Model file for the job. Use its own axes, mm. Face numbers are marked on the shaded views. Coordinates: 2 decimals unless noted, no trailing zeros. Loops run counter-clockwise (first coordinate to the right, second up) from the corner with the lowest first, then second, coordinate; pieces in that order, holes last.
from build123d import *

# Parameters (mm, degrees)
F0_W     = 20
F0_H     = 10.1
F1_DEPTH = 1.5
F2_R     = 1.1
F3_DEPTH = 1.5
F4_R     = 1


with BuildPart() as f1:
    # F0 (on Front) → F1 (new body)
    with BuildSketch(Plane.XZ):
        with Locations((10, 5.05)):
            Rectangle(F0_W, F0_H)
    extrude(amount=F1_DEPTH)

    # F2 (on face) → F3 (cut, through all)
    with BuildSketch(Plane.XZ.offset(1.5)):
        with Locations((2.3, 7.9)):
            Circle(F2_R)
        with Locations((17.7, 7.9)):
            Circle(F2_R)
        with Locations((2.3, 2.2)):
            Circle(F2_R)
        with Locations((17.7, 2.2)):
            Circle(F2_R)
    extrude(amount=-F3_DEPTH, mode=Mode.SUBTRACT)

    # F4
    f4_edges = [f1.edges().sort_by_distance(p)[0] for p in [
        (20, -0.75, 10.1),
        (20, -0.75, 0),
        (0, -0.75, 10.1),
        (0, -0.75, 0),
    ]]
    fillet(f4_edges, radius=F4_R)


solid = f1.part
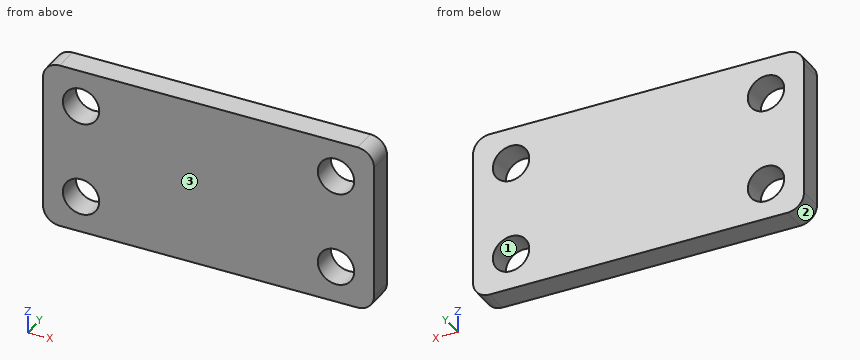
Q1. Slice it at C-C (x = 2.3). List the corners of the cut face in (y, z).
Answers:
outline: (-1.5, 0) - (0, 0) - (0, 1.1) - (-1.5, 1.1) - close; (-1.5, 3.3) - (0, 3.3) - (0, 6.8) - (-1.5, 6.8) - close; (-1.5, 9) - (0, 9) - (0, 10.1) - (-1.5, 10.1) - close
Q2. Slice it at B-B (y = -0.25). List the corners of the cut face in (x, z), and give its area (3 significant figures).
Answers:
outline: (0, 1) arc R1 ccw to (1, 0) - (19, 0) arc R1 ccw to (20, 1) - (20, 9.1) arc R1 ccw to (19, 10.1) - (1, 10.1) arc R1 ccw to (0, 9.1) - close; hole circle Ø2.2 at (2.3, 2.2); hole circle Ø2.2 at (2.3, 7.9); hole circle Ø2.2 at (17.7, 2.2); hole circle Ø2.2 at (17.7, 7.9)
area: 186 mm2
Q3. Mould opens along Z. For the marked faces 1, 2 and 3 say: +Z half, -Z half, draft (parallel to the pull), parting line (faces both ways), or undercut.
Answers:
face 1: undercut
face 2: -Z half
face 3: draft
Q4. Slice it at A-A (z = 2.2). List the corners of the cut face in (x, y), and give its area (3 significant figures).
Answers:
outline: (0, -1.5) - (1.2, -1.5) - (1.2, 0) - (0, 0) - close; (3.4, -1.5) - (16.6, -1.5) - (16.6, 0) - (3.4, 0) - close; (18.8, -1.5) - (20, -1.5) - (20, 0) - (18.8, 0) - close
area: 23.4 mm2
Q5. Flat gauge pin, fed straight in: P1, Ø1.8, axis at x = 2.3, z = 2.2, coming from the +Y side. Where does the tip first touch, or does it go through?
Answers:
P1: passes through
Q6. Drill centre lines: line 1 (Z direction, x = 17.7, y = -1.1); line 2 (Z direction, x = 18.5, y = -0.65); line 3 (X direction, y = -0.6, z = 1.75). Where is each one in solid material? Low to high.
Answers:
line 1: z = 0 to 1.1, 3.3 to 6.8, 9 to 10.1
line 2: z = 0 to 1.45, 2.95 to 7.15, 8.65 to 10.1
line 3: x = 0 to 1.3, 3.3 to 16.7, 18.7 to 20
